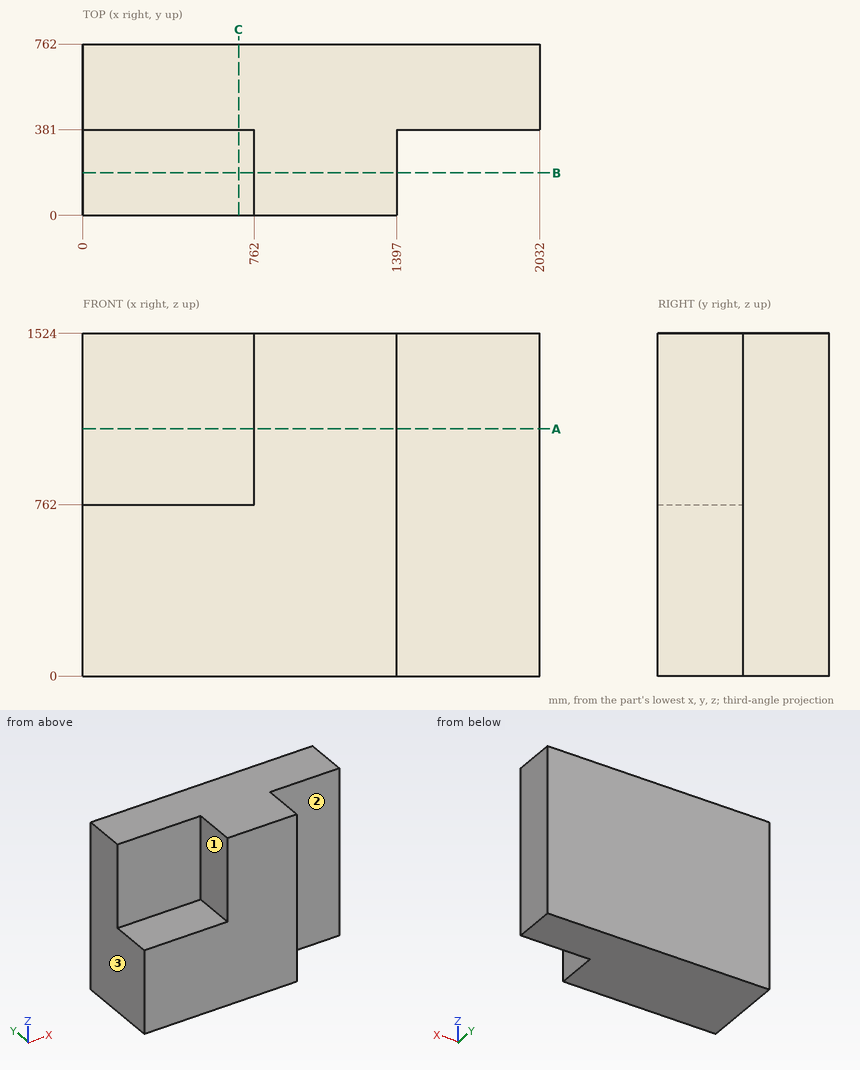
Answer from the drawing. Dimensions are ordinates in mm from the lowest x, y and z of the part. A direction names the side the tool comes from. Round coordinates to 2 decimals unless told otherwise and drop trailing zeros. Loops run counter-clockwise (first coordinate to the right, second up) from the corner with the lowest first, then second, coordinate; pieces in that order, holes last.
Q1. Each of these flat-tipped pins is pushed along its axis until it touches: pin 1 (2 mm diameter, centred on y = 186, z = 305, fed in from +X); pin 2 (12 mm diameter, centred on y = 310, z = 787.5, fed in from -X); pin 3 (8 mm diameter, centred on x = 382.5, z = 1345.5, fed in from -Y). Where does it stop, or does it pass through?
Q2. Section C-C on x = 692.5 is taken. Write down the section's boundary in (y, z).
Q3. Section A-A on z = 1099 is taken. Write down the section's boundary in (x, y).
Q4. Which of the six approach directions +Z, -Z, +X, -X, +Y, -Y give full straight-line access (tool end or side, diameter ignored) to the marked faces 1, 2 and 3?
Q5. Section B-B on y = 188.5 is taken. Write down the section's boundary in (x, z).
Q6. Consider probe 1 along Z at (x, y) = (406, 173); probe 2 along X at (y, z) = (121, 731); probe 3 along Y at (x, z) = (88.5, 1095). Determine where each line is inside the solid, lowest interval first.
Output:
1. pin 1: stops at x = 1397
1. pin 2: stops at x = 762
1. pin 3: stops at y = 381
2. outline: (0, 0) - (762, 0) - (762, 1524) - (381, 1524) - (381, 762) - (0, 762) - close
3. outline: (0, 381) - (762, 381) - (762, 0) - (1397, 0) - (1397, 381) - (2032, 381) - (2032, 762) - (0, 762) - close
4. face 1: +Z, -X, -Y
4. face 2: +Z, -Z, +X, -Y
4. face 3: +Z, -Z, -X, +Y, -Y
5. outline: (0, 0) - (1397, 0) - (1397, 1524) - (762, 1524) - (762, 762) - (0, 762) - close
6. probe 1: z = 0 to 762
6. probe 2: x = 0 to 1397
6. probe 3: y = 381 to 762
